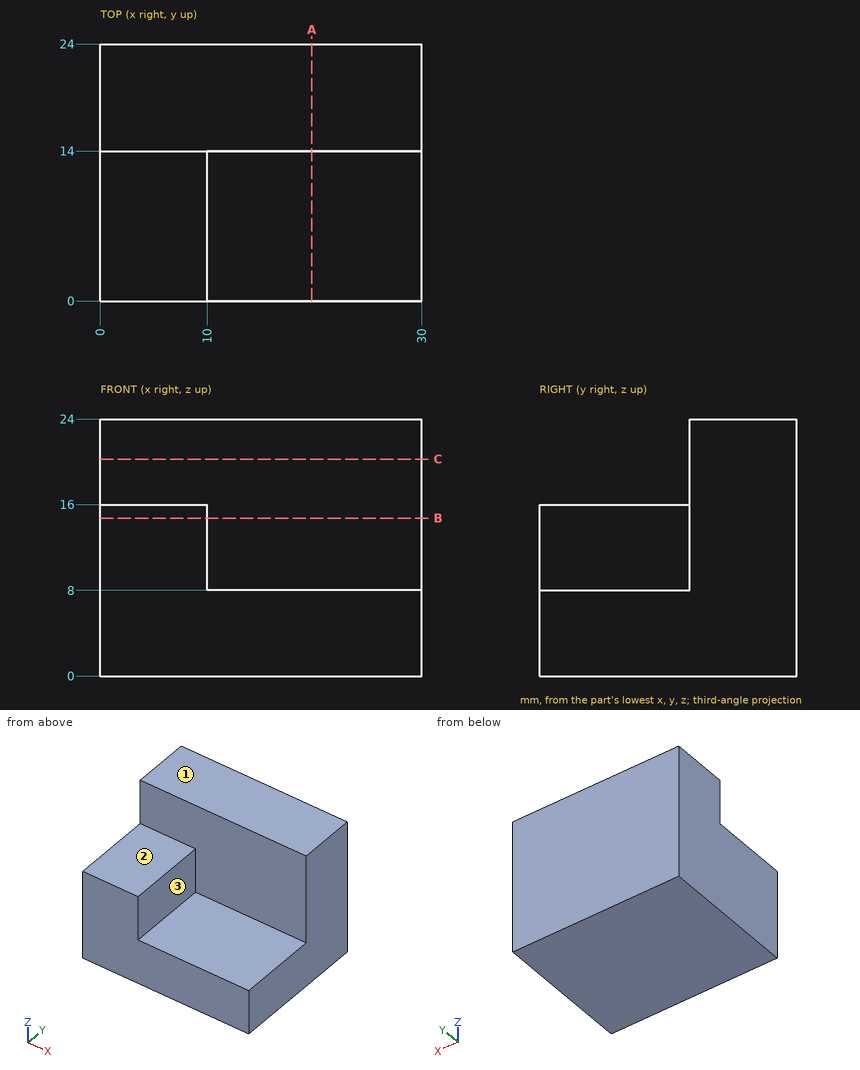
Source: three-view drawing plus pictorial views. Frame: mm from the lowest corner of the part. A direction names the side the tool comes from. Round coordinates to 2 decimals unless told otherwise and drop trailing zeros. Order: outer loops, then holes, each group sorted by start corner. A loop starts at its lowest first (then second) coordinate and runs counter-clockwise, first axis right, second up. Notation, with made-up numbers: (-17, -35.75) - (6, -35.75) arc R16 ccw to (6, -25.75) - close; hole circle Ø5 at (16, 36). An arc over 180 degrees is marked (long way). Answer in a Markdown table with one row per item.
Item 1: Reachability of the marked faces 1, 2 and 3 from +Z, -Z, +X, -X, +Y, -Y: full face, straight path, thin tool, end or side. Return the list, or none.
Model answer:
| item | result |
|---|---|
| face 1 | +Z, +X, -X, +Y, -Y |
| face 2 | +Z, +X, -X, -Y |
| face 3 | +Z, +X, -Y |
Item 2: Section query A-A (x = 19.75). Return the cut outline in (y, z), then the cut area to 3 significant figures.
Model answer:
| item | result |
|---|---|
| outline | (0, 0) - (24, 0) - (24, 24) - (14, 24) - (14, 8) - (0, 8) - close |
| area | 352 mm² |
Item 3: Section query C-C (z = 20.25). Return the cut outline in (x, y), then the cut area to 3 significant figures.
Model answer:
| item | result |
|---|---|
| outline | (0, 14) - (30, 14) - (30, 24) - (0, 24) - close |
| area | 300 mm² |
Item 4: Section query B-B (z = 14.75). Return the cut outline in (x, y), then the cut area to 3 significant figures.
Model answer:
| item | result |
|---|---|
| outline | (0, 0) - (10, 0) - (10, 14) - (30, 14) - (30, 24) - (0, 24) - close |
| area | 440 mm² |
Item 5: Line query: line 1 (X direction, y = 5.5, z = 14.5); line 2 (Z direction, x = 22.5, y = 12.5); line 3 (Y direction, x = 8.5, z = 21.5). Output: solid intervals per line, ascending.
Model answer:
| item | result |
|---|---|
| line 1 | x = 0 to 10 |
| line 2 | z = 0 to 8 |
| line 3 | y = 14 to 24 |
Item 6: Pin query (flat end, axial travel): pin 1 (4 mm diameter, centred on y = 5.5, z = 11, fed in from +X); pin 2 (6 mm diameter, centred on x = 7.5, z = 20.5, fed in from -Y); pin 3 (4 mm diameter, centred on x = 22, y = 10, fed in from +Z). Return the tip coordinate at first contact, or that it passes through.
Model answer:
| item | result |
|---|---|
| pin 1 | stops at x = 10 |
| pin 2 | stops at y = 14 |
| pin 3 | stops at z = 8 |
